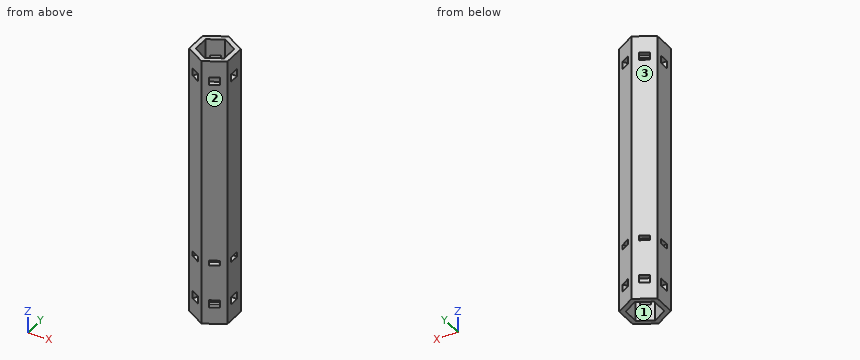
```python
from build123d import *

# Parameters (mm, degrees)
BOSS_EXTRUDE1_DEPTH     = 90
CUT_EXTRUDE2_DEPTH      = 3.175
CUT_EXTRUDE2_DEPTH_BACK = 3.175
SKETCH4_W               = 3.175
SKETCH4_H               = 5
SKETCH4_H_2             = 3.175
CUT_EXTRUDE3_DEPTH      = 3.175
CUT_EXTRUDE3_DEPTH_BACK = 3.175
SKETCH7_W               = 5
SKETCH7_H               = 3.175
SKETCH7_W_2             = 3.175
CUT_EXTRUDE4_DEPTH      = 3.175
CUT_EXTRUDE4_DEPTH_BACK = 3.175
SKETCH8_W               = 5
SKETCH8_H               = 3.175
SKETCH8_W_2             = 3.175


with BuildPart() as part:
    # Sketch3 → Boss-Extrude1 (new, symmetric)
    with BuildSketch(Plane.XY):
        Polygon((0, 14.664696837), (-12.7, 7.332348419), (-12.7, -7.332348419), (0, -14.664696837), (12.7, -7.332348419), (12.7, 7.332348419), align=None)
        Polygon((0, 10.998522628), (9.525, 5.499261314), (9.525, -5.499261314), (0, -10.998522628), (-9.525, -5.499261314), (-9.525, 5.499261314), align=None, mode=Mode.SUBTRACT)
    extrude(amount=BOSS_EXTRUDE1_DEPTH, both=True)

    # Sketch4 → Cut-Extrude2 (cut, two sides: drawn at the far end of the back side and taken through both)
    with BuildSketch(Plane(origin=(0, 0, 0), x_dir=(1, 0, 0), z_dir=(0, 1, 0)).offset(-CUT_EXTRUDE2_DEPTH_BACK)):
        with Locations((-11.1125, -76.325394791)):
            Rectangle(SKETCH4_W, SKETCH4_H)
        with Locations((-11.1125, 48.311416829)):
            Rectangle(SKETCH4_W, SKETCH4_H_2)
        with Locations((11.1125, 76.360728449)):
            Rectangle(SKETCH4_W, SKETCH4_H)
        with Locations((11.1125, 48.311416829)):
            Rectangle(SKETCH4_W, SKETCH4_H_2)
        with Locations((11.1125, -76.325394791)):
            Rectangle(SKETCH4_W, SKETCH4_H)
        with Locations((-11.1125, 76.360728449)):
            Rectangle(SKETCH4_W, SKETCH4_H)
    extrude(amount=CUT_EXTRUDE2_DEPTH + CUT_EXTRUDE2_DEPTH_BACK, mode=Mode.SUBTRACT)

    # Sketch7 → Cut-Extrude3 (cut, two sides: drawn at the far end of the back side and taken through both)
    with BuildSketch(Plane(origin=(0, 0, 0), x_dir=(0, 0, 1), z_dir=(-0.8660254037844387, 0.4999999999999999, 0)).offset(-CUT_EXTRUDE3_DEPTH_BACK)):
        with Locations((76.325394791, -11.1125)):
            Rectangle(SKETCH7_W, SKETCH7_H)
        with Locations((-48.311416829, -11.1125)):
            Rectangle(SKETCH7_W_2, SKETCH7_H)
        with Locations((-76.360728449, 11.1125)):
            Rectangle(SKETCH7_W, SKETCH7_H)
        with Locations((-48.311416829, 11.1125)):
            Rectangle(SKETCH7_W_2, SKETCH7_H)
        with Locations((76.325394791, 11.1125)):
            Rectangle(SKETCH7_W, SKETCH7_H)
        with Locations((-76.360728449, -11.1125)):
            Rectangle(SKETCH7_W, SKETCH7_H)
    extrude(amount=CUT_EXTRUDE3_DEPTH + CUT_EXTRUDE3_DEPTH_BACK, mode=Mode.SUBTRACT)

    # Sketch8 → Cut-Extrude4 (cut, two sides: drawn at the far end of the back side and taken through both)
    with BuildSketch(Plane(origin=(0, 0, 0), x_dir=(0, 0, 1), z_dir=(-0.8660254037844387, -0.4999999999999999, 0)).offset(-CUT_EXTRUDE4_DEPTH_BACK)):
        with Locations((76.325394791, -11.1125)):
            Rectangle(SKETCH8_W, SKETCH8_H)
        with Locations((-48.311416829, -11.1125)):
            Rectangle(SKETCH8_W_2, SKETCH8_H)
        with Locations((-76.360728449, 11.1125)):
            Rectangle(SKETCH8_W, SKETCH8_H)
        with Locations((-48.311416829, 11.1125)):
            Rectangle(SKETCH8_W_2, SKETCH8_H)
        with Locations((76.325394791, 11.1125)):
            Rectangle(SKETCH8_W, SKETCH8_H)
        with Locations((-76.360728449, -11.1125)):
            Rectangle(SKETCH8_W, SKETCH8_H)
    extrude(amount=CUT_EXTRUDE4_DEPTH + CUT_EXTRUDE4_DEPTH_BACK, mode=Mode.SUBTRACT)


solid = part.part
```
Check sheet for the modelled part. Datum: model origin and axes. Units: mm. Face numbers are marked on the shaded views. Round coordinates to 2 decimals unless told otherwise and drop trailing zeros. Order: outer loops, then holes, each group sorted by start corner. A loop starts at its lowest first (then second) coordinate and runs counter-clockwise, first axis right, second up. Notation, with made-up numbers: (60.5, 82.5) - (84.5, 82.5) arc R12 cw to (84.5, 89.5) - close; hole circle Ø1 at (-4.75, -22.5). An arc over 180 degrees is marked (long way). Write item = value, one per line.
Q1. Draft check along Y on the marked faces 1, 2 and 3. Enter one of: pulls with the +Y half, pulls with the -Y half, needs draft (parallel to the pull), parting line crosses it, or undercut.
Computed:
face_1 = undercut
face_2 = pulls with the -Y half
face_3 = pulls with the +Y half
Q2. Section check A-A (z = -23). Record the boundary of the cut face in (x, y) (3 decimals), and give its area (3 significant figures).
Computed:
outline = (-12.7, -7.332) - (0, -14.665) - (12.7, -7.332) - (12.7, 7.332) - (0, 14.665) - (-12.7, 7.332) - close; hole (-9.525, -5.499) - (0, -10.999) - (9.525, -5.499) - (9.525, 5.499) - (0, 10.999) - (-9.525, 5.499) - close
area = 244 mm^2
Q3. Section check B-B (x = 6). State how many separate pieces and enclosed holes the cut face has, and give its area (3 significant figures).
Computed:
separate_pieces = 8
enclosed_holes = 0
area = 1,220 mm^2
Q4. Go/stop test with flat-tipped pins: pin 1 (1 mm diameter, centred on x = 10, z = 55.5, fed in from -Y); pin 2 (1.6 mm diameter, centred on x = -11, z = -49, fed in from +Y); pin 3 (1.6 mm diameter, centred on x = 12, z = 77, fed in from +Y). Record where each tip stops, or that it passes through.
Computed:
pin_1 = -9.18
pin_2 = 8.78
pin_3 = 8.2
Q5. Thickness scan on line 1 along Z through (x, y) = (-4.5, -10.25); line 2 along X through (y, z) = (5.5, 30.5); line 3 along Y through (x, z) = (1.5, -43). Record the ranges inside material, lowest first.
Computed:
line_1 = -90 to -78.86, -73.86 to -49.9, -46.72 to 73.83, 78.83 to 90
line_2 = -12.7 to -9.52, 9.52 to 12.7
line_3 = -13.8 to -10.13, 10.13 to 13.8
